Design review of the part built by this model. Coordinates are the model's own, in mm. A direction names the side the tool comes from. Coordinates: 2 decimals unless noted, no trailing zeros. Loops run counter-clockwise (first coordinate to the right, second up) from the corner with the lowest first, then second, coordinate; pieces in that order, holes last. Notation, with made-up numbers: M 32,-15.75 L 41,-15.75 A31 ccw 41,18.25 Z; hole C 3,20 d3. An arc over 180 degrees is marked long. One line per item, written item: value.
```python
from build123d import *

# Parameters (mm, degrees)
F0_R     = 11
F0_R_2   = 2.5
F1_DEPTH = 48
F2_DEPTH = 2
F3_DEPTH = 24
F4_R     = 2
F5_DEPTH = 5


with BuildPart() as f1:
    # F0 (on Right) → F1 (new body)
    with BuildSketch(Plane.YZ):
        with BuildLine():
            Line((27.518488, 2.104281), (-8.431512, 2.104281))
            ThreePointArc((-8.431512, 2.104281), (-10.676576, 1.174345), (-11.606512, -1.070719))
            Line((-11.606512, -1.070719), (-11.606512, -37.020719))
            ThreePointArc((-11.606512, -37.020719), (-10.676576, -39.265783), (-8.431512, -40.195719))
            Line((-8.431512, -40.195719), (27.518488, -40.195719))
            ThreePointArc((27.518488, -40.195719), (29.763552, -39.265783), (30.693488, -37.020719))
            Line((30.693488, -37.020719), (30.693488, -1.070719))
            ThreePointArc((30.693488, -1.070719), (29.763552, 1.174345), (27.518488, 2.104281))
        make_face()
        with Locations((9.543488, -19.045719)):
            Circle(F0_R, mode=Mode.SUBTRACT)
        with Locations((9.543488, -19.045719)):
            Circle(F0_R)
        with Locations((9.543488, -19.045719)):
            Circle(F0_R_2, mode=Mode.SUBTRACT)
        with Locations((9.543488, -19.045719)):
            Circle(F0_R_2)
    extrude(amount=F1_DEPTH)

    # F0 (on Right) → F2 (join)
    with BuildSketch(Plane.YZ):
        with Locations((9.543488, -19.045719)):
            Circle(F0_R)
        with Locations((9.543488, -19.045719)):
            Circle(F0_R_2, mode=Mode.SUBTRACT)
        with Locations((9.543488, -19.045719)):
            Circle(F0_R_2)
    extrude(amount=-F2_DEPTH)

    # F0 (on Right) → F3 (join)
    with BuildSketch(Plane.YZ):
        with Locations((9.543488, -19.045719)):
            Circle(F0_R_2)
    extrude(amount=-F3_DEPTH)

    # F4 (on face) → F5 (cut)
    with BuildSketch(Plane.YZ):
        with BuildLine():
            ThreePointArc((25.043488, -5.545719), (26.457701, -4.959933), (27.043488, -3.545719))
            ThreePointArc((27.043488, -3.545719), (25.043488, -1.545719), (23.043488, -3.545719))
            Line((23.043488, -3.545719), (25.043488, -3.545719))
            Line((25.043488, -3.545719), (25.043488, -5.545719))
        make_face()
        with BuildLine():
            Line((25.043488, -3.545719), (23.043488, -3.545719))
            ThreePointArc((23.043488, -3.545719), (23.629274, -4.959933), (25.043488, -5.545719))
            Line((25.043488, -5.545719), (25.043488, -3.545719))
        make_face()
        with BuildLine():
            ThreePointArc((27.043488, -34.545719), (26.457701, -33.131506), (25.043488, -32.545719))
            Line((25.043488, -32.545719), (25.043488, -34.545719))
            Line((25.043488, -34.545719), (23.043488, -34.545719))
            ThreePointArc((23.043488, -34.545719), (25.043488, -36.545719), (27.043488, -34.545719))
        make_face()
        with BuildLine():
            Line((25.043488, -34.545719), (25.043488, -32.545719))
            ThreePointArc((25.043488, -32.545719), (23.629274, -33.131506), (23.043488, -34.545719))
            Line((23.043488, -34.545719), (25.043488, -34.545719))
        make_face()
        with Locations((-5.956512, -34.545719)):
            Circle(F4_R)
        with Locations((-5.956512, -3.545719)):
            Circle(F4_R)
    extrude(amount=F5_DEPTH, mode=Mode.SUBTRACT)


solid = f1.part
```
(1) We need section C-C on z = -28.5. State the section outline as (x, y) points, then the cut area to 3 significant figures.
Reply:
outline: M -2,3.92 L 0,3.92 L 0,-11.61 L 48,-11.61 L 48,30.69 L 0,30.69 L 0,15.17 L -2,15.17 Z
area: 2,050 mm2
(2) Mouldability with a two-part tool opening along Y and no side actions: class faces 3 (the flat face through (-24, 10, -19)), 4 (the cylindrical face through (2.465, -7.955, -3.458)), 5 (the flat face through (24, 30.693, -19)) as released by +Y, released by -Y, zero draft, split by the parting line, or undercut.
Reply:
face 3: zero draft
face 4: undercut
face 5: released by +Y
(3) Insertion check: pin 1 (12 mm diameter, centred on y = -3, z = -13.5, fed in from -X); pin 2 (6.5 mm diameter, centred on y = 4.5, z = -16.5, fed in from -X); pin 3 (2 mm diameter, centred on y = 25, z = -35, fed in from -X); pin 4 (3 mm diameter, centred on y = -5.5, z = -4, fed in from -X). Each pin has a flat end and moves straight along its axis. Give the tip position at first contact, or say it passes through.
Reply:
pin 1: stops at x = -2
pin 2: stops at x = -24
pin 3: stops at x = 5
pin 4: stops at x = 0
(4) To check wall thickness, follow line 1 along X through (y, z) = (5, -32); line 2 along Y through (x, z) = (26, -1); line 3 along X through (y, z) = (7, -12.5). State the ranges of each line that lie inside material, in increasing order. Write a range as [from, to].
Reply:
line 1: x = [0, 48]
line 2: y = [-11.61, 30.69]
line 3: x = [-2, 48]
(5) Tool access review of faces 1 (the flat face through (0, 19, -28)), 2 (the cylindrical face through (23.66, 29.79, 1.15)): name each direction out of +Z, -Z, +X, -X, +Y, -Y from which nothing blocks a thin tool from reaching the whole face with its end or side.
Reply:
face 1: -X
face 2: +Z, +X, -X, +Y
(6) We need section B-B on y = 16. State the section outline as (x, z) points, then the cut area to 3 significant figures.
Reply:
outline: M -2,-27.95 L 0,-27.95 L 0,-40.2 L 48,-40.2 L 48,2.1 L 0,2.1 L 0,-10.14 L -2,-10.14 Z
area: 2,070 mm2
(7) We need section D-D on y = -6. State the section outline as (x, z) points.
Reply:
outline: M 0,-40.2 L 48,-40.2 L 48,2.1 L 0,2.1 L 0,-1.55 L 5,-1.55 L 5,-5.55 L 0,-5.55 L 0,-32.55 L 5,-32.55 L 5,-36.55 L 0,-36.55 Z
(8) We need section A-A on x = 2. State the section outline as (y, z) points (3 decimals).
Reply:
outline: M -11.607,-37.021 A3.175 ccw -8.432,-40.196 L 27.518,-40.196 A3.175 ccw 30.693,-37.021 L 30.693,-1.071 A3.175 ccw 27.518,2.104 L -8.432,2.104 A3.175 ccw -11.607,-1.071 Z; hole C -5.957,-34.546 d4; hole C -5.957,-3.546 d4; hole M 23.043,-3.546 A2 ccw 25.043,-5.546 A2 ccw long Z; hole M 25.043,-32.546 A2 ccw long 27.043,-34.546 A2 ccw Z
